from build123d import *

# Parameters (mm, degrees)
PAD_DEPTH       = 5
POCKET003_DEPTH = 3
SKETCH011_R     = 1.5
POCKET004_DEPTH = 10


with BuildPart() as part:
    # Sketch009 (on Face5 of Pad002) → Pad (new body)
    with BuildSketch(Plane(origin=(0, 0, 0), x_dir=(1, 0, 0), z_dir=(0, 0, -1))):
        Polygon((-64.221279, 23.538714), (-71.221279, 23.538714), (-71.221279, -22.461286), (-64.221279, -22.461286), (-64.221279, -29.461286), (121.778721, -29.461286), (121.778721, -22.461286), (128.778721, -22.461286), (128.778721, 23.538714), (121.778721, 23.538714), (121.778721, 30.538714), (-64.221279, 30.538714), align=None)
    extrude(amount=PAD_DEPTH)

    # Sketch010 (on Face13 of Pad) → Pocket003 (cut)
    with BuildSketch(Plane.XY):
        Polygon((-61.721279, -28.038714), (-61.721279, -21.038714), (-68.721279, -21.038714), (-68.721279, 19.961286), (-61.721279, 19.961286), (-61.721279, 26.961286), (119.278721, 26.961286), (119.278721, 19.961286), (126.278721, 19.961286), (126.278721, -21.038714), (119.278721, -21.038714), (119.278721, -28.038714), align=None)
    extrude(amount=-POCKET003_DEPTH, mode=Mode.SUBTRACT)

    # Sketch011 (on Face27 of Pocket003) → Pocket004 (cut)
    with BuildSketch(Plane.XY.offset(-3)):
        with Locations((-48.657681, 23.169219)):
            Circle(SKETCH011_R)
        with Locations((-34.114651, 7.669219)):
            Circle(SKETCH011_R)
        with Locations((26.342319, 22.86806)):
            Circle(SKETCH011_R)
        with Locations((-25.157681, -20.330781)):
            Circle(SKETCH011_R)
        with Locations((-56.157681, -25.330781)):
            Circle(SKETCH011_R)
        with Locations((26.342319, -25.63194)):
            Circle(SKETCH011_R)
        with Locations((52.5, -11.63194)):
            Circle(SKETCH011_R)
        with Locations((52.5, -16.63194)):
            Circle(SKETCH011_R)
        with Locations((73, 18.059744)):
            Circle(SKETCH011_R)
        with Locations((73, -20.940256)):
            Circle(SKETCH011_R)
    extrude(amount=-POCKET004_DEPTH, mode=Mode.SUBTRACT)


solid = part.part
Build history of the part. All positions in model axes, mm. A direction names the side the tool comes from. Coordinates: 2 decimals unless noted, no trailing zeros. Order: outer loops, then holes, each group sorted by start corner. A loop starts at its lowest first (then second) coordinate and runs counter-clockwise, first axis right, second up. Notation, with made-up numbers: (17, 21.5) -> (47, 21.5) arc R33 ccw to (47, 58.5) -> close; hole circle Ø2 at (-26.5, 5). An arc over 180 degrees is marked (long way). One line per item, written item: value.
(1) Probe line 1 (X direction, y = -28, z = -0.8); line 2 (Y direction, x = 74, z = -0.75); line 3 (X direction, y = -11.5, z = -1.4). List the from-to ranges inside material, lowest first. Write a range as [from, to].
Checked values:
line 1: [-64.22, -61.72], [119.28, 121.78]
line 2: [-30.54, -28.04], [26.96, 29.46]
line 3: [-71.22, -68.72], [126.28, 128.78]
(2) Slice it at A-A, the plane z = -1.9. List the corners of the cut face in (x, y), plus the area to 4 significant figures.
Checked values:
outline: (-71.22, -23.54) -> (-64.22, -23.54) -> (-64.22, -30.54) -> (121.78, -30.54) -> (121.78, -23.54) -> (128.78, -23.54) -> (128.78, 22.46) -> (121.78, 22.46) -> (121.78, 29.46) -> (-64.22, 29.46) -> (-64.22, 22.46) -> (-71.22, 22.46) -> close; hole (-68.72, -21.04) -> (-61.72, -21.04) -> (-61.72, -28.04) -> (119.28, -28.04) -> (119.28, -21.04) -> (126.28, -21.04) -> (126.28, 19.96) -> (119.28, 19.96) -> (119.28, 26.96) -> (-61.72, 26.96) -> (-61.72, 19.96) -> (-68.72, 19.96) -> close
area: 1,275 mm2
(3) Mould opens along X. For faces 6 (the flat face through (125, 22.461, -2)), 7 (the flat face through (121.779, 26, -2)), 8 (the flat face through (30, 0, -3)), 9 (the flat face through (-64.221, 26, -2)) say: pulls with the +X half, pulls with the -X half, needs draft (parallel to the pull), parting line crosses it, or undercut.
Checked values:
face 6: needs draft
face 7: pulls with the +X half
face 8: undercut
face 9: pulls with the -X half
(4) Tool access for faces 1 (the flat face through (27, -1, -5)), 2 (the flat face through (-64.221, -27, -2)), 3 (the flat face through (30, -30.539, -2)), 4 (the flat face through (125, -23.539, -2)), 5 (the flat face through (-68, 22.461, -2)): list every direction of +Z, -Z, +X, -X, +Y, -Y with a clear straight run to the whole face (end or side of a thin tool).
Checked values:
face 1: -Z, +X, -X, +Y, -Y
face 2: +Z, -Z, -X, -Y
face 3: +Z, -Z, +X, -X, -Y
face 4: +Z, -Z, +X, -Y
face 5: +Z, -Z, -X, +Y
(5) Drop flat-ended pins along their axis: pin 1 Ø4 at (x, y) = (78.5, -13.5) entering from +Z; pin 2 Ø2.5 at (x, z) = (-66, -1.5) entering from +Y. Give the stop position or say it passes through.
Checked values:
pin 1: z = -3
pin 2: y = 22.46
(6) Slice it at C-C, the plane y = -2. List the corners of the cut face in (x, z).
Checked values:
outline: (-71.22, -5) -> (128.78, -5) -> (128.78, 0) -> (126.28, 0) -> (126.28, -3) -> (-68.72, -3) -> (-68.72, 0) -> (-71.22, 0) -> close
(7) Slice it at B-B, the plane x = 49. List the corners of the cut face in (y, z), plus the area to 3 significant figures.
Checked values:
outline: (-30.54, -5) -> (29.46, -5) -> (29.46, 0) -> (26.96, 0) -> (26.96, -3) -> (-28.04, -3) -> (-28.04, 0) -> (-30.54, 0) -> close
area: 135 mm2
